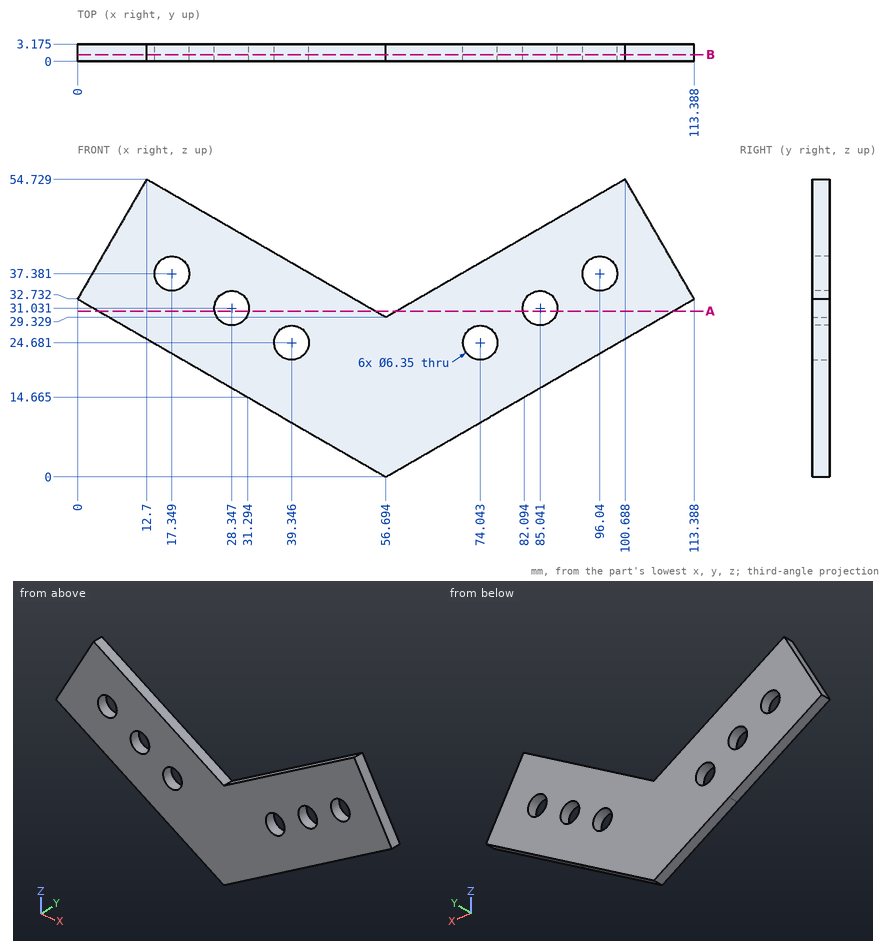
Answer from the drawing. Dimensions are ordinates in mm from the lowest x, y and z of the part. Give positions to 0.01 mm unless a question says otherwise; leave off trailing zeros. Order: outer loops, then holes, each group sorted by start corner. A loop starts at its lowest first (then second) coordinate and runs counter-clockwise, first axis right, second up.
Item 1: Find the intervals of material crossed by probe 1 along X at (y, z) = (0.8, 26) (1 decimal); probe 2 along X at (y, z) = (2.4, 39.5) (1 decimal); probe 3 along Z at (x, y) = (19, 2.55), in increasing order.
From the geometry:
probe 1: x = 11.7 to 36.5, 42.2 to 71.2, 76.9 to 101.7
probe 2: x = 3.9 to 15, 19.7 to 39.1, 74.3 to 93.7, 98.4 to 109.5
probe 3: z = 21.76 to 34.67, 40.09 to 51.09
Item 2: The part is cut by section B-B, the plane y = 1.2. Count the separate pieces of the cut face and the enclosed holes in it, and give its area (3 significant figures).
From the geometry:
separate pieces: 1
enclosed holes: 6
area: 2,760 mm2
Item 3: The part is cut by section A-A, the plane z = 30.5. Give the vertices of the cut face in (x, y) (1 decimal).
From the geometry:
outline: (3.9, 0) - (25.2, 0) - (25.2, 3.2) - (3.9, 3.2) - close; (31.5, 0) - (54.7, 0) - (54.7, 3.2) - (31.5, 3.2) - close; (58.7, 0) - (81.9, 0) - (81.9, 3.2) - (58.7, 3.2) - close; (88.2, 0) - (109.5, 0) - (109.5, 3.2) - (88.2, 3.2) - close
Item 4: Given pin 1 Ø7.5 at (x, z) = (17.35, 37.38) entering from -Y; pin 2 Ø1.5 at (y, z) = (0.5, 28.5) entering from -X, each flat-ended and moving along its own axis, determine where each tip first touches the part or whether it passes through.
From the geometry:
pin 1: stops at y = 0
pin 2: stops at x = 6.03
